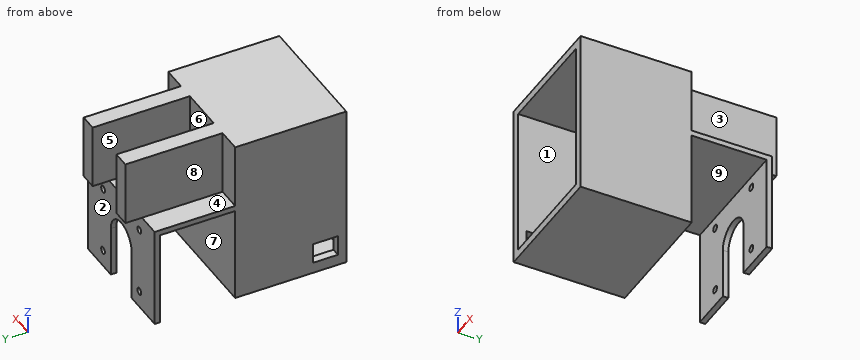
from build123d import *

# Parameters (mm, degrees)
SKETCH3_W                         = 57.15
SKETCH3_H                         = 76.2
BOSS_EXTRUDE2_DEPTH               = 50.8
SKETCH4_W                         = 49.53
SKETCH4_H                         = 68.58
CUT_EXTRUDE2_DEPTH                = 44.45
CUT_EXTRUDE3_REACH                = 109.95
SKETCH5_W                         = 9.398
SKETCH5_H                         = 11.43
MOTOR_MOUNTING_SHAPE_DEPTH        = 57.15
MOTOR_MOUNTING_HOLES_REACH        = 131.428
SKETCH8_R                         = 1.6
SKETCH7_W                         = 7.62
SKETCH7_H                         = 29.66
TRAY_SUPPORT_MOUNTING_SHAPE_DEPTH = 44.45


with BuildPart() as part:
    # Sketch3 → Boss-Extrude2 (new body)
    with BuildSketch(Plane(origin=(0, 0, 0), x_dir=(-1, 0, 0), z_dir=(0, 1, 0))):
        with Locations((28.575, 38.1)):
            Rectangle(SKETCH3_W, SKETCH3_H)
    extrude(amount=-BOSS_EXTRUDE2_DEPTH)

    # Sketch4 → Cut-Extrude2 (cut)
    with BuildSketch(Plane.XZ.offset(50.8)):
        with Locations((-28.575, 38.1)):
            Rectangle(SKETCH4_W, SKETCH4_H)
    extrude(amount=-CUT_EXTRUDE2_DEPTH, mode=Mode.SUBTRACT)

    # Sketch5 → Cut-Extrude3 (cut, up to next)
    with BuildSketch(Plane(origin=(-57.15, 0, 0), x_dir=(0, 0, -1), z_dir=(1, 0, 0)), mode=Mode.PRIVATE) as cut_extrude3_sk1:
        with Locations((-9.779, -41.275)):
            Rectangle(SKETCH5_W, SKETCH5_H)
    cut_extrude3_tool1 = extrude(cut_extrude3_sk1.sketch, amount=CUT_EXTRUDE3_REACH, mode=Mode.PRIVATE) & part.part
    add(cut_extrude3_tool1.solids().sort_by_distance((-57.15, -41.275, 9.779))[0], mode=Mode.SUBTRACT)

    # Sketch6 → Motor Mounting Shape (add)
    with BuildSketch(Plane.ZY.offset(57.15)):
        Polygon((46.54, 0), (46.54, 36.83), (0, 36.83), (0, 34.29), (44, 34.29), (44, 0), align=None)
    extrude(amount=-MOTOR_MOUNTING_SHAPE_DEPTH)

    # Sketch8 → Motor-Mounting-Holes (cut, up to next)
    with BuildSketch(Plane(origin=(0, 36.83, 0), x_dir=(1, 0, 0), z_dir=(0, 1, 0)), mode=Mode.PRIVATE) as motor_mounting_holes_sk1:
        with Locations(Location((-44.075, -7.77, 0), (0, 0, 270))):
            Circle(SKETCH8_R)
    motor_mounting_holes_tool1 = extrude(motor_mounting_holes_sk1.sketch, amount=-MOTOR_MOUNTING_HOLES_REACH, mode=Mode.PRIVATE) & part.part
    # Sketch8 → Motor-Mounting-Holes (cut, up to next)
    with BuildSketch(Plane(origin=(0, 36.83, 0), x_dir=(1, 0, 0), z_dir=(0, 1, 0)), mode=Mode.PRIVATE) as motor_mounting_holes_sk2:
        with Locations(Location((-13.075, -7.77, 0), (0, 0, 270))):
            Circle(SKETCH8_R)
    motor_mounting_holes_tool2 = extrude(motor_mounting_holes_sk2.sketch, amount=-MOTOR_MOUNTING_HOLES_REACH, mode=Mode.PRIVATE) & part.part
    # Sketch8 → Motor-Mounting-Holes (cut, up to next)
    with BuildSketch(Plane(origin=(0, 36.83, 0), x_dir=(1, 0, 0), z_dir=(0, 1, 0)), mode=Mode.PRIVATE) as motor_mounting_holes_sk3:
        with Locations(Location((-13.075, -38.77, 0), (0, 0, 270))):
            Circle(SKETCH8_R)
    motor_mounting_holes_tool3 = extrude(motor_mounting_holes_sk3.sketch, amount=-MOTOR_MOUNTING_HOLES_REACH, mode=Mode.PRIVATE) & part.part
    # Sketch8 → Motor-Mounting-Holes (cut, up to next)
    with BuildSketch(Plane(origin=(0, 36.83, 0), x_dir=(1, 0, 0), z_dir=(0, 1, 0)), mode=Mode.PRIVATE) as motor_mounting_holes_sk4:
        with Locations(Location((-44.075, -38.77, 0), (0, 0, 270))):
            Circle(SKETCH8_R)
    motor_mounting_holes_tool4 = extrude(motor_mounting_holes_sk4.sketch, amount=-MOTOR_MOUNTING_HOLES_REACH, mode=Mode.PRIVATE) & part.part
    # Sketch8 → Motor-Mounting-Holes (cut, up to next)
    with BuildSketch(Plane(origin=(0, 36.83, 0), x_dir=(1, 0, 0), z_dir=(0, 1, 0)), mode=Mode.PRIVATE) as motor_mounting_holes_sk5:
        with BuildLine():
            Line((-37.465, 0), (-19.685, 0))
            Line((-19.685, 0), (-19.685, -23.27))
            ThreePointArc((-19.685, -23.27), (-28.575, -32.16), (-37.465, -23.27))
            Line((-37.465, -23.27), (-37.465, 0))
        make_face()
    motor_mounting_holes_tool5 = extrude(motor_mounting_holes_sk5.sketch, amount=-MOTOR_MOUNTING_HOLES_REACH, mode=Mode.PRIVATE) & part.part
    add(motor_mounting_holes_tool1.solids().sort_by_distance((-44.075, 36.83, 7.77))[0], mode=Mode.SUBTRACT)
    add(motor_mounting_holes_tool2.solids().sort_by_distance((-13.075, 36.83, 7.77))[0], mode=Mode.SUBTRACT)
    add(motor_mounting_holes_tool3.solids().sort_by_distance((-13.075, 36.83, 38.77))[0], mode=Mode.SUBTRACT)
    add(motor_mounting_holes_tool4.solids().sort_by_distance((-44.075, 36.83, 38.77))[0], mode=Mode.SUBTRACT)
    add(motor_mounting_holes_tool5.solids().sort_by_distance((-28.575, 36.83, 15.191166))[0], mode=Mode.SUBTRACT)

    # Sketch7 → Tray Support Mounting Shape (add)
    with BuildSketch(Plane(origin=(0, 0, 0), x_dir=(1, 0, 0), z_dir=(0, 1, 0))):
        with Locations((-42.545, -61.37)):
            Rectangle(SKETCH7_W, SKETCH7_H)
        with Locations((-14.605, -61.37)):
            Rectangle(SKETCH7_W, SKETCH7_H)
    extrude(amount=TRAY_SUPPORT_MOUNTING_SHAPE_DEPTH)


solid = part.part
Verification items for the finished model (mm, model axes). Face numbers are marked on the shaded views. A direction names the side the tool comes from. Coordinates: 2 decimals unless noted, no trailing zeros. Order: outer loops, then holes, each group sorted by start corner. A loop starts at its lowest first (then second) coordinate and runs counter-clockwise, first axis right, second up. Notation, with made-up numbers: (80.5, 18) -> (86.5, 18) arc R13 ccw to (86.5, 43) -> close; hole circle Ø10 at (9.5, -40). An arc over 180 degrees is marked (long way). Put each result on its own line as item: value. Start each with the question number.
1. Material ranges on L1, parallel to X at y = 36.35, z = 38.77 (3 decimals); L2, parallel to X at y = -11, z = 39.5; L3, parallel to Y at x = -38, z = 14, recorded low to high. Write a range as [from, to].
2. Access from +Z, -Z, +X, -X, +Y, -Y to the whole of each face (thin tool, end or side, straight path). Record for the marked faces 1, 2, 3, 4 and 5.
3. Mould release check, pull along Y, two halves, no side actions. Record for the marked faces 6, 7, 8 and 9: released by +Y, released by -Y, zero draft, split by the parting line, or undercut.
4. Go/stop test with flat-tipped pins: pin 1 Ø1.1 at (x, z) = (-55.5, 9) entering from +Y; pin 2 Ø17 at (x, y) = (-42.5, 17.5) entering from -Z; pin 3 Ø5 at (x, z) = (-21, 35.5) entering from -Y. Record where each tip stops, or that it passes through.
5. Cross-section at D-D, the plane y = 25. Record the boundary of the cut face in (x, z) (3 decimals), then the cut area to 3 significant figures.
6. Cross-section at A-A, the plane z = 33.5. Record the boundary of the cut face in (x, y).
7. Cross-section at C-C, the plane z = 7.77. Record the boundary of the cut face in (x, y) (3 decimals), then the cut area to 3 significant figures.
8. Cross-section at B-B, the plane x = -50.5. Record the boundary of the cut face in (y, z).
Computed:
1. L1: [-57.15, -45.675], [-42.475, -14.675], [-11.475, 0]
1. L2: [-57.15, -53.34], [-3.81, 0]
1. L3: [-6.35, 0], [34.29, 36.83]
2. face 1: -Y
2. face 2: -Z, +X, -X, +Y
2. face 3: +Z, +X, +Y
2. face 4: +Z, -X, +Y
2. face 5: +Z, +Y
3. face 6: released by +Y
3. face 7: undercut
3. face 8: zero draft
3. face 9: undercut
4. pin 1: y = 36.83
4. pin 2: z = 44
4. pin 3: y = -6.35
5. outline: (-57.15, 44) -> (0, 44) -> (0, 46.54) -> (-10.795, 46.54) -> (-10.795, 76.2) -> (-18.415, 76.2) -> (-18.415, 46.54) -> (-38.735, 46.54) -> (-38.735, 76.2) -> (-46.355, 76.2) -> (-46.355, 46.54) -> (-57.15, 46.54) -> close
5. area: 597 mm2
6. outline: (-57.15, -50.8) -> (-53.34, -50.8) -> (-53.34, -6.35) -> (-3.81, -6.35) -> (-3.81, -50.8) -> (0, -50.8) -> (0, 0) -> (-57.15, 0) -> close; (-57.15, 34.29) -> (0, 34.29) -> (0, 36.83) -> (-57.15, 36.83) -> close
7. outline: (-57.15, -50.8) -> (-53.34, -50.8) -> (-53.34, -46.99) -> (-57.15, -46.99) -> close; (-57.15, -35.56) -> (-53.34, -35.56) -> (-53.34, -6.35) -> (-3.81, -6.35) -> (-3.81, -50.8) -> (0, -50.8) -> (0, 0) -> (-57.15, 0) -> close; (-57.15, 34.29) -> (-45.675, 34.29) -> (-45.675, 36.83) -> (-57.15, 36.83) -> close; (-42.475, 34.29) -> (-37.465, 34.29) -> (-37.465, 36.83) -> (-42.475, 36.83) -> close; (-19.685, 34.29) -> (-14.675, 34.29) -> (-14.675, 36.83) -> (-19.685, 36.83) -> close; (-11.475, 34.29) -> (0, 34.29) -> (0, 36.83) -> (-11.475, 36.83) -> close
7. area: 742 mm2
8. outline: (-50.8, 0) -> (0, 0) -> (0, 44) -> (34.29, 44) -> (34.29, 0) -> (36.83, 0) -> (36.83, 46.54) -> (0, 46.54) -> (0, 76.2) -> (-50.8, 76.2) -> (-50.8, 72.39) -> (-6.35, 72.39) -> (-6.35, 3.81) -> (-50.8, 3.81) -> close
